Source: CAD feature listing. Evaluate the final solid. Frame: model axes, mm. Face numbers are marked on the shaded views. A direction names the side the tool comes from. Coordinates: 2 decimals unless noted, no trailing zeros. Write each loop counter-clockwise with the first axis right and the second up, starting at its lowest first coordinate (ties: lowest second). Pieces come first, ordered by that corner, then holes. Notation, with made-up numbers: M 65,32.25 L 96,32.25 A15 cw 96,54.25 Z; hole C 42.5,27.25 d5. An arc over 180 degrees is marked long. Write item = value, one per line. Start each with the question number.
1. Line query: line 1 along Z through (x, y) = (2, 23.75); line 2 along Y through (x, z) = (-1, 6.5); line 3 along X through (y, z) = (32.5, 9). Output: solid intervals per line, ascending.
2. Section query D-D (y = 29). Output: boundary loops of the cut face in (x, z), then the cut area to 3 significant figures.
3. Section query A-A (x = -1). Output: boundary loops of the cut face in (y, z), then the cut area to 3 significant figures.
4. Pull-direction query (Y, two-part tool) for the marked faces 1, 2 and 3; classes: pulls with the +Y half, pulls with the -Y half, needs draft (parallel to the pull), parting line crosses it, or undercut.
5. Section query C-C (y = 16). Output: boundary loops of the cut face in (x, z), then the cut area to 3 significant figures.
6. Access query for the marked faces 4 and 5. Directions: +Z, -Z, +X, -X, +Y, -Y. A direction counts if a zero-diameter tool reaches every point of the face in a straight line with its end or side. Return the directions, or none.
7. Section query B-B (z = 3). Output: boundary loops of the cut face in (x, y), then the cut area to 3 significant figures.
8. Pin query (flat end, axial travel): pin 1 Ø0.6 at (y, z) = (17, 11) entering from -X; pin 2 Ø4 at (x, z) = (-1.5, 6.5) entering from +Y; pin 3 Ø1.5 at (x, y) = (-1, 32.5) entering from +Z; pin 4 Ø2 at (x, y) = (1, 21.5) entering from -Z. Return the tip coordinate at first contact, or that it passes through.
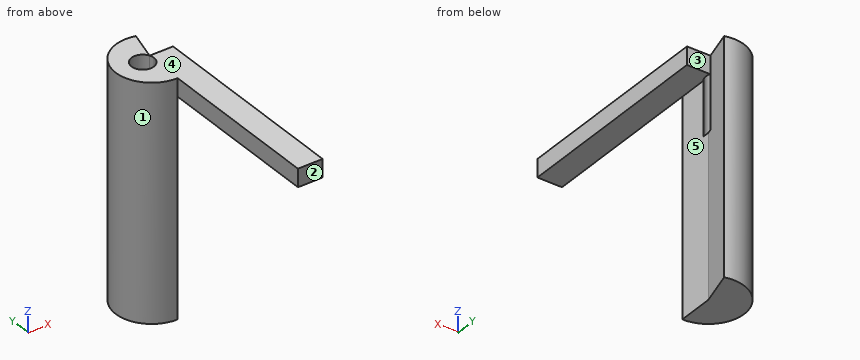
```python
from build123d import *

# Parameters (mm, degrees)
CYLINDER006_R               = 1.25
CYLINDER006_DEPTH           = 10
BOX004_W                    = 23
BOX004_H                    = 2.75
BOX004_DEPTH                = 2
CYLINDER001_W               = 4
CYLINDER001_H               = 26
CYLINDER001_ANGLE           = 195
CYLINDER001_PLACEMENT_ANGLE = 75


with BuildPart() as obj1:
    # Cylinder006 → Cylinder006 (new body)
    with BuildSketch(Plane(origin=(-1, 12.5, 4), x_dir=(1, 0, 0), z_dir=(0, 0, 1))):
        Circle(CYLINDER006_R)
    extrude(amount=CYLINDER006_DEPTH)


with BuildPart() as w012:
    # Box004 → Box004 (new body)
    with BuildSketch(Plane(origin=(2.75, -10, 10), x_dir=(0, 1, 0), z_dir=(0, 0, 1))):
        with Locations((11.5, 1.375)):
            Rectangle(BOX004_W, BOX004_H)
    extrude(amount=BOX004_DEPTH)


with BuildPart() as cut003_w:
    # Cylinder001 → Cylinder001 (revolve)
    with BuildSketch(Plane.XZ):
        with Locations((2, 13)):
            Rectangle(CYLINDER001_W, CYLINDER001_H)
    revolve(axis=Axis((0, 0, 0), (0, 0, 1)), revolution_arc=CYLINDER001_ANGLE)


with BuildPart() as cut003_w_1:
    # Cylinder001 placement: moved
    add(cut003_w.part.moved(Location((0, 12.5, -14))).rotate(Axis((0, 12.5, -14), (0, 0, 1)), CYLINDER001_PLACEMENT_ANGLE))

    # Fusion003: union W012
    add(w012.part)

    # Cut003: cut obj1
    add(obj1.part, mode=Mode.SUBTRACT)


with BuildPart() as cut003_w_2:
    # Cut003 placement: moved
    add(cut003_w_1.part.moved(Location((0, 20, 0))))


solid = cut003_w_2.part
```
Results are:
q1.line_1 = 10 to 12
q1.line_2 = 28.63 to 31.25, 33.75 to 36.37
q1.line_3 = -4 to -2.25
q2.outline = M -1.94,-14 L 0,-14 L 0,10 L 2.75,10 L 2.75,12 L -1.94,12 Z
q2.area = 55.8 mm^2
q3.outline = M 28.63,-14 L 36.37,-14 L 36.37,12 L 33.75,12 L 33.75,4 L 31.25,4 L 31.25,12 L 28.63,12 Z
q3.area = 181 mm^2
q4.face_1 = parting line crosses it
q4.face_2 = pulls with the -Y half
q4.face_3 = undercut
q5.outline = M 0,10 L 2.75,10 L 2.75,12 L 0,12 Z
q5.area = 5.50 mm^2
q6.face_4 = +Z, +X, -X, +Y, -Y
q6.face_5 = -Z, +X, -Y
q7.outline = M 0,28.5 L 0,32.5 L 1.04,36.36 A4 ccw long Z
q7.area = 27.2 mm^2
q8.pin_1 = 0
q8.pin_2 = 36.5
q8.pin_3 = 4
q8.pin_4 = 10
